Source: CAD feature listing. Evaluate the final solid. Frame: model axes, mm. A direction names the side the tool comes from. Coordinates: 2 decimals unless noted, no trailing zeros. Loops run counter-clockwise (first coordinate to the right, second up) from the corner with the lowest first, then second, coordinate; pieces in that order, holes last.
Item 1: Section query C-C, the plane z = 34.5. Return the cut outline in (x, y) (3 decimals).
Item 2: Section query A-A, the plane z = 17. Return the cut outline in (x, y) (3 decimals), then the cut area to 3 significant figures.
Item 3: Pull-direction query (X, two-part tool) for faces 5 (the flat face through (-25.311, 6.644, 49.787)), 6 (the flat face through (-13, -3.41, 49)), 7 (the flat face through (3.175, -1, 13)); classes: +X half, -X half, draft (parallel to the pull), parting line (faces both ways), or undercut.
Item 4: Reachability of faces 1 (the flat face through (-30.14, 0.125, 19.442)), 2 (the flat face through (0, -1, 13)), 3 (the flat face through (-12, -5, 45.551)), 4 (the flat face through (4.74, -0.449, 19.536)) from +Z, -Z, +X, -X, +Y, -Y: full face, straight path, thin tool, end or side. Return the list, or none.
Item 5: Line query: probe 1 along X at (y, z) = (14, 13.5) (3 decimals); probe 2 along X at (y, z) = (15, 38.5); probe 3 along Z at (x, y) = (-12.7, -15.9). Output: solid intervals per line, ascending.
Item 6: Pin query (flat end, axial travel): pin 1 Ø2 at (x, z) = (-26, 12) entering from -Y; pin 2 Ø6 at (y, z) = (-4.5, 10.5) entering from +X (3 decimals); pin 3 Ø1.1 at (x, y) = (-31.5, 14) entering from -Z. Return the tip coordinate at first contact, or that it passes through.
Autodesk Inventor part; units mm, degrees
ref_plane "YZ Plane Vertical Spine" through (0, 0, 0) normal (1, 0, 0) x (0, 1, 0)
ref_plane "XZ Plane Horizontal" through (0, 0, 0) normal (0, 1, 0) x (-1, 0, 0)
ref_plane "XY Plane Vertical Span" through (0, 0, 0) normal (0, 0, 1) x (1, 0, 0)
sketch "Sketch1" plane through (0, 0, 0) normal (1, 0, 0) x (0, 1, 0)
  circle A0 centre (9.6489, 11.4476) radius 2.4892
  line L0 (2.3561, 6.2073) -> (18.2812, 3.5994)
  line L1 (33.7025, 135.9395) -> (135.3025, 135.9395) construction
  line L2 (21.99, 26.2473) -> (-14.84, 26.2473)
  line L3 (4.4085, 18.7403) -> (-20.6576, 22.8451)
  line L4 (-20.6576, 22.8451) -> (-22.71, 10.312)
  line L5 (-22.71, 10.312) -> (2.3561, 6.2073)
  circle A1 centre (-15.4173, 15.5524) radius 2.4892
  line L6 (-14.84, 26.2473) -> (-14.84, 46.5673)
  line L7 (-20.6576, 22.8451) -> (-16.7225, 46.8756)
  line L8 (-16.7225, 46.8756) -> (-14.84, 46.5673)
  line L9 (21.99, 26.2473) -> (18.2812, 3.5994)
  line L10 (20.3336, 16.1325) -> (4.4085, 18.7403)
  dimension "d11" = 12.7
  dimension "d13" = 4.9784
  dimension "d14" = 20.32
extrude "Extrusion1" add sketch "Sketch1" along normal blind 3.175
sketch "Sketch2" plane through (0, 0, 0) normal (-1, 0, 0) x (0, 0, 1)
  line L0 (26.2473, 21.99) -> (26.2473, -14.84)
  line L1 (3.5994, 18.2812) -> (26.2473, 21.99)
  line L2 (26.2473, -14.84) -> (46.5673, -14.84)
  line L3 (46.8756, -16.7225) -> (10.312, -22.71)
  line L4 (16.1325, 20.3336) -> (22.8451, -20.6576)
  line L5 (16.1325, 20.3336) -> (26.2473, 21.99)
  line L6 (26.2473, 21.5334) -> (26.2473, -14.84)
  line L7 (26.2473, -14.84) -> (46.5673, -14.84)
  line L8 (46.5673, -14.84) -> (46.8756, -16.7225)
  line L9 (46.8756, -16.7225) -> (22.8451, -20.6576)
extrude "Extrusion2" add sketch "Sketch2" along normal blind 25.4
sketch "Sketch3" plane through (-25.4, 0, 0) normal (-1, 0, 0) x (0, 0, 1)
  line L0 (26.2473, -14.84) -> (26.2473, 21.99)
  line L1 (3.5994, 18.2812) -> (16.1325, 20.3336)
  line L2 (26.2473, 21.99) -> (16.1325, 20.3336)
  line L3 (46.5673, -14.84) -> (26.2473, -14.84)
  line L4 (46.8756, -16.7225) -> (46.5673, -14.84)
  line L5 (22.8451, -20.6576) -> (46.8756, -16.7225)
  line L6 (22.8451, -20.6576) -> (10.312, -22.71)
  line L7 (10.312, -22.71) -> (3.5994, 18.2812)
  circle A0 centre (15.5524, -15.4173) radius 2.4892
  circle A1 centre (11.4476, 9.6489) radius 2.4892
extrude "Extrusion3" add sketch "Sketch3" along normal blind 3.175
sketch "Sketch4" plane through (-28.575, 0, 0) normal (-1, 0, 0) x (0, 0, 1)
  line L0 (26.2473, 21.99) -> (3.5994, 18.2812)
  line L1 (26.2473, -14.84) -> (26.2473, 21.99)
  line L2 (46.5673, -14.84) -> (26.2473, -14.84)
  line L3 (46.8756, -16.7225) -> (46.5673, -14.84)
  line L4 (10.312, -22.71) -> (46.8756, -16.7225)
  line L5 (46.8756, -16.7225) -> (46.5673, -14.84)
  line L6 (46.5673, -14.84) -> (26.2473, -14.84)
  line L7 (26.2473, -14.84) -> (26.2473, 21.99)
  line L8 (26.2473, 21.99) -> (3.5994, 18.2812)
  line L9 (3.5994, 18.2812) -> (10.312, -22.71)
  line L10 (10.312, -22.71) -> (46.8756, -16.7225)
  circle A0 centre (11.4476, 9.6489) radius 2.4892
  circle A1 centre (15.5524, -15.4173) radius 2.4892
  line L11 (16.1325, 20.3336) -> (22.8451, -20.6576)
  line L12 (16.1325, 20.3336) -> (26.2473, 21.99)
  line L13 (26.2473, 21.99) -> (26.2473, -14.84)
  line L14 (46.5673, -14.84) -> (26.2473, -14.84)
  line L15 (46.5673, -14.84) -> (46.8756, -16.7225)
  line L16 (46.8756, -16.7225) -> (22.8451, -20.6576)
extrude "Extrusion4" add sketch "Sketch4" along normal blind 3.175 contours L1 L2 L3 L4 L11 L0
sketch "Sketch5" plane through (3.175, 0, 0) normal (1, 0, 0) x (0, 0, -1)
  line L0 (-22.8451, -20.6576) -> (-16.1325, 20.3336)
  line L1 (-46.8756, -16.7225) -> (-10.312, -22.71)
  line L2 (-26.2473, -14.84) -> (-46.5673, -14.84)
  line L3 (-26.2473, 21.99) -> (-26.2473, -14.84)
  line L4 (-3.5994, 18.2812) -> (-26.2473, 21.99)
  line L5 (-26.2473, 21.99) -> (-16.1325, 20.3336)
  line L6 (-16.1325, 20.3336) -> (-22.8451, -20.6576)
  line L7 (-22.8451, -20.6576) -> (-46.8756, -16.7225)
  line L8 (-46.8756, -16.7225) -> (-46.5673, -14.84)
  line L9 (-46.5673, -14.84) -> (-26.2473, -14.84)
  line L10 (-26.2473, -14.84) -> (-26.2473, 21.99)
extrude "Extrusion5" add sketch "Sketch5" along normal blind 3.175
sketch "Sketch6" plane through (-31.75, -14.84, 46.5673) normal (0, 1, 0) x (1, 0, 0)
  line L0 (38.1, 20.32) -> (38.1, 0)
  line L1 (0, 0) -> (0, 20.32)
  line L2 (0, 20.32) -> (1.27, 20.32)
  line L3 (0, 0) -> (1.27, 0)
  line L4 (1.27, 0) -> (1.27, 20.32)
  line L5 (38.1, 0) -> (38.1, 20.32)
  line L6 (38.1, 20.32) -> (36.83, 20.32)
  line L7 (36.83, 20.32) -> (36.83, 0)
  line L8 (36.83, 0) -> (38.1, 0)
  dimension "d24" = 1.27
  dimension "d25" = 1.27
  dimension "d26" = 1.27
extrude "Extrusion6" add sketch "Sketch6" along normal blind 36.83
sketch "Sketch7" plane through (-30.48, -14.84, 26.2473) normal (0, 1, 0) x (1, 0, 0)
  line L0 (0, -20.32) -> (35.56, -20.32)
  line L1 (0, -19.05) -> (35.56, -19.05)
  line L2 (0, -20.32) -> (35.56, -20.32)
  line L3 (35.56, -19.05) -> (35.56, -20.32)
  line L4 (0, -19.05) -> (0, -20.32)
  dimension "d29" = 1.27
extrude "Extrusion7" add sketch "Sketch7" along normal blind 11.43
sketch "Sketch8" plane through (-30.48, -14.84, 26.2473) normal (1, 0, 0) x (0, 0, -1)
  line L0 (-20.32, 11.43) -> (-20.32, 36.83)
  line L1 (-19.05, 11.43) -> (-19.05, 36.83)
  line L2 (-19.05, 36.83) -> (-20.32, 36.83)
  line L3 (-19.05, 11.43) -> (-20.32, 11.43)
  line L4 (-20.32, 11.43) -> (-20.32, 36.83)
  dimension "d32" = 1.27
extrude "Extrusion8" add sketch "Sketch8" along normal blind 11.43
sketch "Sketch9" plane through (5.08, -14.84, 26.2473) normal (-1, 0, 0) x (0, 0, 1)
  line L0 (20.32, 11.43) -> (20.32, 36.83)
  line L1 (19.0567, 11.43) -> (19.0567, 36.83)
  line L2 (19.0567, 36.83) -> (20.32, 36.83)
  line L3 (20.32, 36.83) -> (20.32, 11.43)
  line L4 (20.32, 11.43) -> (19.0567, 11.43)
extrude "Extrusion9" add sketch "Sketch9" along normal blind 11.43
sketch "Sketch10" plane through (-31.75, 0, 0) normal (-1, 0, 0) x (0, 0, 1)
  line L0 (46.5673, -14.84) -> (46.5673, 21.99)
  line L1 (22.8451, -20.6576) -> (46.8756, -16.7225)
  line L2 (46.5673, -14.84) -> (46.5673, -16.773)
  line L3 (46.5673, -16.773) -> (47.6603, -17.0438)
  line L4 (47.6603, -17.0438) -> (46.5673, -14.84)
extrude "Extrusion10" cut sketch "Sketch10" against normal blind 50.8
thicken "Thicken1" operation add thickness 6.35 both sides no extend neighbours no toward (0, 0, 1) faces at (-10.5833, -12.3187, 46.5673)
sketch "Sketch11" plane through (-31.75, 0, 0) normal (-1, 0, 0) x (0, 0, 1)
  line L0 (22.8451, -20.6576) -> (46.5673, -16.773)
  line L1 (46.5673, -16.773) -> (55.5301, -15.3053)
  line L2 (55.5301, -15.3053) -> (55.5301, -20.6762)
  line L3 (55.5301, -20.6762) -> (46.5673, -16.773)
extrude "Extrusion11" cut sketch "Sketch11" against normal blind 50.8
chamfer "Chamfer1" distance 6.35 distance2 12.7 1 edges at (-31.75, 3.1284, 52.9173) measured on face at (-31.75, -4.8003, 34.0032)
chamfer "Chamfer2" distance 6.35 distance2 12.7 1 edges at (6.35, 3.1284, 52.9173) measured on face at (6.35, -4.8003, 34.0032)
chamfer "Chamfer3" distance 6.35 distance2 12.319 1 edges at (-12.7, -15.7331, 52.9173) measured on face at (-14.8167, -19.0161, 32.8692)
sketch "Sketch13" plane through (-31.75, 0, 0) normal (-1, 0, 0) x (0, 0, 1)
  line L0 (26.2473, 21.99) -> (46.5673, 21.99)
  line L1 (37.0423, 21.99) -> (33.8673, 21.99)
  line L2 (30.6923, 21.99) -> (30.6923, 4.21)
  line L3 (37.0423, 4.21) -> (37.0423, 21.99)
  line L4 (37.0423, 21.99) -> (30.6923, 21.99)
  arc A0 (30.6923, 4.21) -> (37.0423, 4.21) centre (33.8673, 4.21) ccw
  point P0 (30.6923, 4.21)
extrude "Extrusion12" cut sketch "Sketch13" against normal blind 25.4
sketch "Sketch14" plane through (-30.48, -14.84, 26.2473) normal (0, 1, 0) x (1, 0, 0)
  line L0 (0, -19.05) -> (35.56, -19.05)
  line L1 (35.56, -19.05) -> (35.56, 0)
  line L2 (0, 0) -> (35.56, 0)
  line L3 (0, 0) -> (0, -19.05)
  line L4 (35.814, 0.254) -> (35.814, -19.304)
  line L5 (35.814, -19.304) -> (-0.254, -19.304)
  line L6 (-0.254, -19.304) -> (-0.254, 0.254)
  line L7 (-0.254, 0.254) -> (35.814, 0.254)
  dimension "d57" = 0.254
extrude "Extrusion13" cut sketch "Sketch14" along normal blind 50.8 contours L3 L2 L1 L0 | L4 L5 L6 L7
sketch "Sketch15" plane through (-30.734, -14.84, 45.5513) normal (0, 1, 0) x (1, 0, 0)
  line L0 (0, 19.558) -> (0, 0)
  line L1 (0, 0) -> (36.068, 0)
  line L2 (36.068, 0) -> (36.068, 19.558)
  line L3 (36.068, 19.558) -> (0, 19.558)
  line L4 (0, 9.779) -> (36.068, 9.779)
  line L5 (18.034, 0) -> (18.034, 19.558)
  circle A0 centre (18.034, 9.779) radius 6.35
  dimension "d60" = 12.7
extrude "Extrusion14" cut sketch "Sketch15" against normal blind 50.8 contours A0 L5 L4 | L4 L5 A0 | A0 L4 L5 | L4 A0 L5
properties part number "back_mount_3DPrint"
Verdict:
1. outline: (-31.75, -18.749) - (-28.575, -18.749) - (-18.921, -18.749) - (-18.921, -14.84) - (-30.734, -14.84) - (-30.734, 1.099) - (-31.75, 1.099) - close; (-6.479, -18.749) - (3.175, -18.749) - (6.35, -18.749) - (6.35, 21.99) - (5.334, 21.99) - (5.334, -14.84) - (-6.479, -14.84) - close
2. outline: (-31.75, 15.036) - (-28.575, 15.036) - (-28.575, -13.392) - (-25.4, -13.392) - (-25.4, 15.036) - (0, 15.036) - (0, -13.392) - (3.175, -13.392) - (3.175, 15.036) - (6.35, 15.036) - (6.35, 20.476) - (-28.575, 20.476) - (-31.75, 20.476) - close; (-28.575, -21.615) - (-25.4, -21.615) - (-25.4, -17.442) - (-28.575, -17.442) - close; (0, -21.615) - (3.175, -21.615) - (3.175, -17.442) - (0, -17.442) - close
2. area: 414 mm2
3. face 5: -X half
3. face 6: undercut
3. face 7: +X half
4. face 1: -Z, -X, -Y
4. face 2: -Z, -Y
4. face 3: +Y
4. face 4: -Z, +X, -Y
5. probe 1: x = -28.575 to -25.4, 0 to 3.175
5. probe 2: x = -31.75 to -30.73, 5.33 to 6.35
5. probe 3: z = 22.07 to 29.42, 42.12 to 47.05
6. pin 1: stops at y = -22.6
6. pin 2: stops at x = 3.175
6. pin 3: stops at z = 17.08
